Geometry check sheet. Reference: drawing and pictorial views, mm from the part's lowest x, y, z. Give positions to 0.01 mm unless a question says otherwise; leave off trailing zeros. Write each loop counter-clockwise with the first axis right and the second up, starting at its lowest first coordinate (ties: lowest second). Pieces come first, ordered by that corner, then holes. Notation, with made-up numbers: M 79.5,83 L 89.5,83 A4 ccw 89.5,90 Z; hole C -4,26.25 d7. An arc over 180 degrees is marked long. Write item = value, one per line. Start each with the question number.
1) Cross-section at D-D, the plane y = 14. Record the cut outline in (x, z).
2) Cross-section at B-B, the plane y = 40. Record the cut outline in (x, z).
3) Go/stop test with flat-tipped pins: pin 1 (5.5 mm diameter, centred on y = 70.5, z = 7.5, fed in from +X); pin 2 (6 mm diameter, centred on x = 8, z = 8.5, fed in from +Y); pin 3 (8 mm diameter, centred on x = 20.5, y = 35, fed in from +Z); pin 4 (1 mm diameter, centred on x = 39.5, z = 5, fed in from +Y). Record where each tip stops, or that it passes through.
4) Scan lines: line 1 along Z through (x, y) = (46.95, 10); line 2 along Z through (x, y) = (44, 25.5); line 3 along Y through (x, z) = (45, 8). Record each from-to range of solid material in increasing order. Write a range as [from, to].
5) Cross-section at C-C, the plane x = 9.5. Record the cut outline in (y, z).
6) Cross-section at A-A, the plane z = 4. Record the cut outline in (x, y), plus the area to 3 significant figures.
7) Mould release check, pull along Y, two halves, no side actions. Record for the marked faces 1, 2, 3 and 4: released by +Y, released by -Y, zero draft, split by the parting line, or undercut.
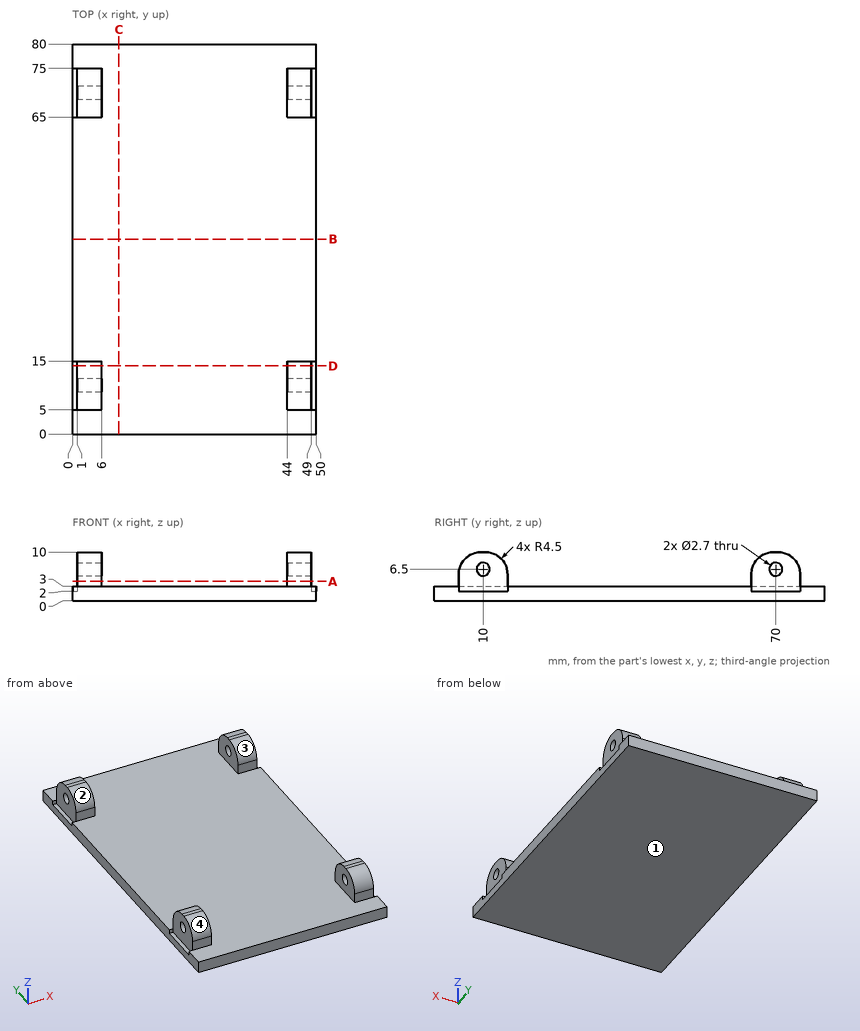
Reply:
q1.outline = M 0,0 L 50,0 L 50,2 L 49,2 L 49,8.33 L 44,8.33 L 44,3 L 6,3 L 6,8.33 L 1,8.33 L 1,2 L 0,2 Z
q2.outline = M 0,0 L 50,0 L 50,3 L 0,3 Z
q3.pin_1 = 49
q3.pin_2 = 74.93
q3.pin_3 = 3
q3.pin_4 = through
q4.line_1 = [0, 5.15], [7.85, 10]
q4.line_2 = [0, 3]
q4.line_3 = [5.76, 14.24], [65.76, 74.24]
q5.outline = M 0,0 L 80,0 L 80,3 L 0,3 Z
q6.outline = M 1,5 L 6,5 L 6,15 L 1,15 Z; M 1,65 L 6,65 L 6,75 L 1,75 Z; M 44,5 L 49,5 L 49,15 L 44,15 Z; M 44,65 L 49,65 L 49,75 L 44,75 Z
q6.area = 200 mm2
q7.face_1 = zero draft
q7.face_2 = undercut
q7.face_3 = undercut
q7.face_4 = released by -Y
